For this review, use the dimensioned drawing (mm, ordinates from the lowest corner) and the shaded views. A direction names the side the tool comes from. Give positions to 0.01 mm unless a question says otherwise; leave off trailing zeros. Order: outer loops, then holes, each group sorted by start corner. A loop starts at its lowest first (then second) coordinate and runs counter-clockwise, first axis right, second up.
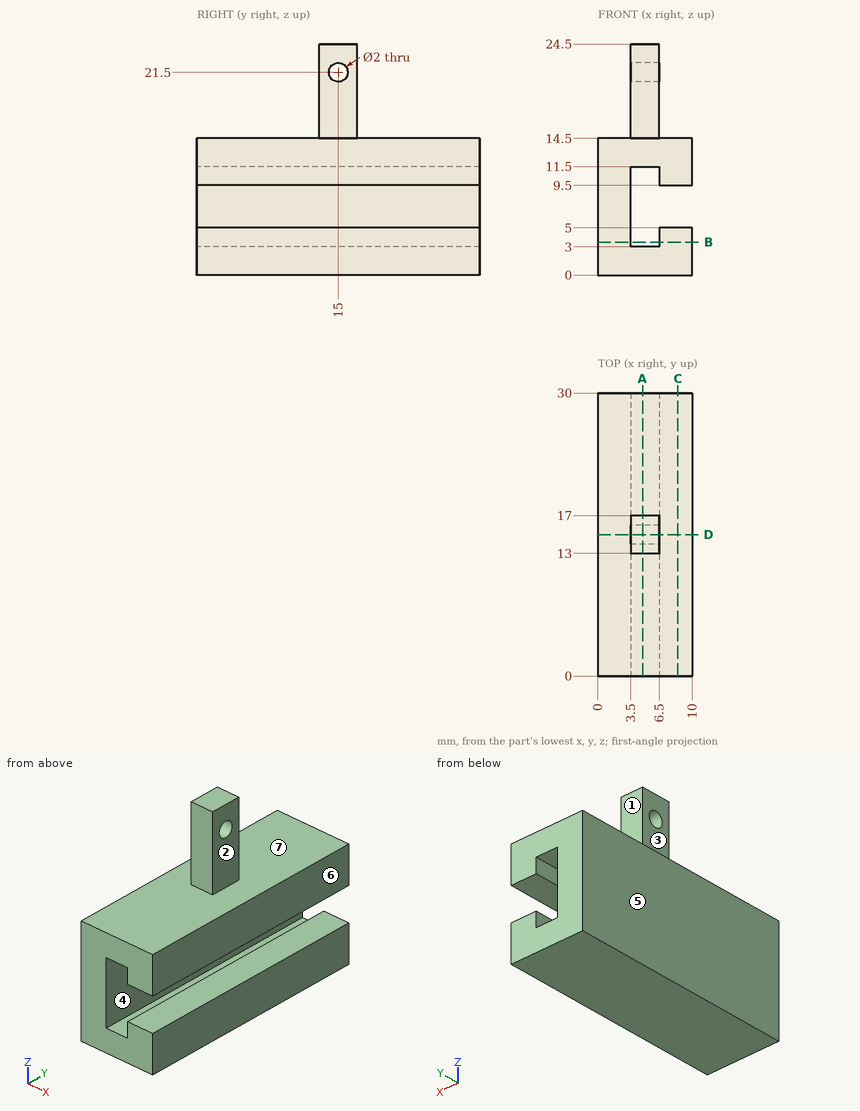
1. Machinability: for the marked faces 1, 2 and 3, which of the approach directions +Z, -Z, +X, -X, +Y, -Y give a long, thin tool a straight path to every point of the face, cutting with its end or side? Answer none if there is none.
Recorded:
face 1: +Z, +X, -X, +Y
face 2: +Z, +X, +Y, -Y
face 3: +Z, -X, +Y, -Y
2. Draft analysis for pull direction X (two halves, no side actions). For the marked faces 4, 5, 6 and 7, state which applies: pulls with the +X half, pulls with the -X half, needs draft (parallel to the pull), parting line crosses it, or undercut.
Recorded:
face 4: undercut
face 5: pulls with the -X half
face 6: pulls with the +X half
face 7: needs draft
3. For line 1 along Z through (x, y) = (4.15, 15); line 2 along Z through (x, y) = (5.25, 11); line 3 along Z through (x, y) = (2.5, 27.5), list the stretches that pass through material, from the lowest coordinate up.
Recorded:
line 1: z = 0 to 3, 11.5 to 20.5, 22.5 to 24.5
line 2: z = 0 to 3, 11.5 to 14.5
line 3: z = 0 to 14.5
4. For pin 1 (4 mm diameter, centred on y = 9.5, z = 22, fed in from +X); pin 2 (7 mm diameter, centred on y = 16, z = 7.5, fed in from +X); pin 3 (1.2 mm diameter, centred on y = 15, z = 17.5, fed in from -X); pin 4 (3 mm diameter, centred on y = 16, z = 19, fed in from +X), all flat-tipped, find the tip position at first contact; note any pin that passes through.
Recorded:
pin 1: passes through
pin 2: stops at x = 10
pin 3: stops at x = 3.5
pin 4: stops at x = 6.5
5. Take a section at B-B (z = 3.5). State the section outline as (x, y) points.
Recorded:
outline: (0, 0) - (3.5, 0) - (3.5, 30) - (0, 30) - close; (6.5, 0) - (10, 0) - (10, 30) - (6.5, 30) - close
6. Take a section at A-A (x = 4.75). State the section outline as (y, z) points, then the cut area to 3 significant figures.
Recorded:
outline: (0, 0) - (30, 0) - (30, 3) - (0, 3) - close; (0, 11.5) - (30, 11.5) - (30, 14.5) - (17, 14.5) - (17, 24.5) - (13, 24.5) - (13, 14.5) - (0, 14.5) - close; hole circle Ø2 at (15, 21.5)
area: 217 mm2
7. Take a section at C-C (x = 8.5). State the section outline as (y, z) points, then the cut area to 3 significant figures.
Recorded:
outline: (0, 0) - (30, 0) - (30, 5) - (0, 5) - close; (0, 9.5) - (30, 9.5) - (30, 14.5) - (0, 14.5) - close
area: 300 mm2
8. Take a section at D-D (y = 15). State the section outline as (x, z) points.
Recorded:
outline: (0, 0) - (10, 0) - (10, 5) - (6.5, 5) - (6.5, 3) - (3.5, 3) - (3.5, 11.5) - (6.5, 11.5) - (6.5, 9.5) - (10, 9.5) - (10, 14.5) - (6.5, 14.5) - (6.5, 20.5) - (3.5, 20.5) - (3.5, 14.5) - (0, 14.5) - close; (3.5, 22.5) - (6.5, 22.5) - (6.5, 24.5) - (3.5, 24.5) - close
